Source: CAD feature listing. Evaluate the final solid. Frame: model axes, mm. A direction names the side the tool comes from. Round coordinates to 2 decimals unless told otherwise and drop trailing zeros. Loops run counter-clockwise (first coordinate to the right, second up) from the corner with the lowest first, then second, coordinate; pieces in that order, holes last. Notation, with made-up numbers: (13.25, 3.5) -> (71.25, 3.5) arc R30 cw to (71.25, 28.5) -> close; hole circle Ø10 at (85.25, 74.25). An arc over 180 degrees is marked (long way). Put each result on its own line as item: value. Start each with the question number.
1. Contact query for flat-ended pins moving along their axis: pin 1 (3.5 mm diameter, centred on x = -10.5, y = -1.5, fed in from +Z); pin 2 (4 mm diameter, centred on y = 5.5, z = 5.5, fed in from +X); pin 3 (1.5 mm diameter, centred on y = 3, z = 4.5, fed in from +X). Output: stop coordinate, or through.
2. Cut plane A-A (x = 13). Return the cut outline in (y, z), then the cut area to 3 significant figures.
3. Draft query along Y for faces 3 (the flat face through (0, -10, 1)), 4 (the flat face through (-13, 0, 7)), 5 (the flat face through (0, 10, 1)), 6 (the flat face through (13, 6.5, 8)). Return one class per face: pulls with the +Y half, pulls with the -Y half, needs draft (parallel to the pull), parting line crosses it, or undercut.
4. Cut plane B-B (y = 0). Return the cut outline in (x, z), then the cut area to 3 significant figures.
5. Set-up query: faces 1 (the flat face through (-22.5, 0, 1)), 2 (the cylindrical face through (-6.94, 1.88, 7.51)). Return all of +Z, -Z, +X, -X, +Y, -Y with unobstructed straight access to the full face (end or side cutting, diameter ignored); none if empty.
6. Material intervals for L1, parallel to X at y = -3.5, z = 7.5; L2, parallel to X at y = -2.5, z = 4; L3, parallel to Y at x = -12.9, z = 7.6, sorted ascending.
```python
from build123d import *

# Parameters (mm, degrees)
SKETCH_1_R          = 8.25
SKETCH_1_W          = 45
SKETCH_1_H          = 20
EXTRUDE_1_DEPTH     = 3
SKETCH_1_3_R        = 8.25
EXTRUDE_2_DEPTH     = 8
SKETCH_2_R          = 6.25
CUT_EXTRUDE_1_DEPTH = 1
FILLET_1_R          = 1


with BuildPart() as part:
    # Sketch 1 → Extrude 1 (new body)
    with BuildSketch(Plane.XY):
        with Locations((-12.9, 0)):
            Circle(SKETCH_1_R)
        with Locations((13, 0)):
            Circle(SKETCH_1_R)
        Rectangle(SKETCH_1_W, SKETCH_1_H)
        with Locations((13, 0)):
            Circle(SKETCH_1_R, mode=Mode.SUBTRACT)
        with Locations((-12.9, 0)):
            Circle(SKETCH_1_R, mode=Mode.SUBTRACT)
    extrude(amount=EXTRUDE_1_DEPTH)

    # Sketch 1_3 → Extrude 2 (add)
    with BuildSketch(Plane.XY):
        with Locations((-12.9, 0)):
            Circle(SKETCH_1_3_R)
        with Locations((13, 0)):
            Circle(SKETCH_1_3_R)
    extrude(amount=EXTRUDE_2_DEPTH)

    # Sketch 2 → Cut-Extrude 1 (cut)
    with BuildSketch(Plane.XY.offset(8)):
        with Locations((13, 0)):
            Circle(SKETCH_2_R)
        with Locations((-12.9, 0)):
            Circle(SKETCH_2_R)
    extrude(amount=-CUT_EXTRUDE_1_DEPTH, mode=Mode.SUBTRACT)

    # Fillet 1
    fillet_1_edges = [part.edges().sort_by_distance(p)[0] for p in [
        (-21.15, 0, 3),
        (-21.15, 0, 8),
        (4.75, 0, 3),
        (4.75, 0, 8),
    ]]
    fillet(fillet_1_edges, radius=FILLET_1_R)


solid = part.part
```
Solution:
1. pin 1: stops at z = 7
1. pin 2: stops at x = 20.47
1. pin 3: stops at x = 20.94
2. outline: (-10, 0) -> (10, 0) -> (10, 3) -> (9.25, 3) arc R1 cw to (8.25, 4) -> (8.25, 7) arc R1 ccw to (7.25, 8) -> (6.25, 8) -> (6.25, 7) -> (-6.25, 7) -> (-6.25, 8) -> (-7.25, 8) arc R1 ccw to (-8.25, 7) -> (-8.25, 4) arc R1 cw to (-9.25, 3) -> (-10, 3) -> close
2. area: 130 mm^2
3. face 3: pulls with the -Y half
3. face 4: undercut
3. face 5: pulls with the +Y half
3. face 6: needs draft
4. outline: (-22.5, 0) -> (22.5, 0) -> (22.5, 3) -> (22.25, 3) arc R1 cw to (21.25, 4) -> (21.25, 7) arc R1 ccw to (20.25, 8) -> (19.25, 8) -> (19.25, 7) -> (6.75, 7) -> (6.75, 8) -> (5.75, 8) arc R1 ccw to (4.75, 7) -> (4.75, 4) arc R1 cw to (3.75, 3) -> (-3.65, 3) arc R1 cw to (-4.65, 4) -> (-4.65, 7) arc R1 ccw to (-5.65, 8) -> (-6.65, 8) -> (-6.65, 7) -> (-19.15, 7) -> (-19.15, 8) -> (-20.15, 8) arc R1 ccw to (-21.15, 7) -> (-21.15, 4) arc R1 cw to (-22.15, 3) -> (-22.5, 3) -> close
4. area: 275 mm^2
5. face 1: +Z, -Z, -X, +Y, -Y
5. face 2: +Z
6. L1: x = -20.22 to -18.08, -7.72 to -5.58, 5.68 to 7.82, 18.18 to 20.32
6. L2: x = -20.76 to -5.04, 5.14 to 20.86
6. L3: y = -8.05 to -6.25, 6.25 to 8.05
